The listing builds one solid part. Answer for the finished solid, in the listing's coordinates (mm). A direction names the side the tool comes from. Give positions to 0.01 mm unless a question says otherwise; leave off trailing zeros. Loops run counter-clockwise (first coordinate to the right, second up) from the corner with the lowest first, then second, coordinate; pieces in that order, holes last. Notation, with made-up numbers: (-9, -20.75) - (21, -20.75) arc R16 ccw to (21, -6.75) - close; hole circle Ø1 at (42.5, 42.5). An arc over 180 degrees is marked (long way). One line per item, written item: value. Start each with the question number.
Autodesk Fusion 360 part; units mm, degrees
sketch "Sketch1" plane through (0, 0, 0) normal (0, 0, 1) x (1, 0, 0)
  circle A0 centre (0, 0) radius 10
  dimension "d1" = 20
extrude "Extrude1" add sketch "Sketch1" along normal blind 3
sketch "Sketch2" plane through (0, 0, 3) normal (0, 0, 1) x (-1, 0, 0)
  circle A0 centre (0, 0) radius 10
  line L0 (-4.2, 1.3) -> (4.2, 1.3)
  line L1 (4.2, 1.3) -> (4.2, -1.3)
  line L2 (4.2, -1.3) -> (-4.2, -1.3)
  line L3 (-4.2, -1.3) -> (-4.2, 1.3)
  line L4 (-4.2, 1.3) -> (4.2, -1.3) construction
  line L5 (4.2, 1.3) -> (-4.2, -1.3) construction
  dimension "d4" = 8.4
  dimension "d5" = 2.6
extrude "Extrude2" cut sketch "Sketch2" against normal blind 6 contours L0 L1 L2 L3
fillet "Fillet1" radius 1.3 4 edges at (4.2, 1.3, 1.5) (4.2, -1.3, 1.5) (-4.2, 1.3, 1.5) (-4.2, -1.3, 1.5)
extrude "Extrude3" add 1 faces at (-0.2491, -4.1907, 3) along direction (0, 0, 1) blind 1
hole "Hole1" at (10, 0, 2.0667) direction (-1, 0, 0) diameter 2 depth 4 tip angle 180
mirror "Mirror1" about plane through (0, 0, 0) normal (1, 0, 0) of "Hole1"
1. A cutting plane is placed at D-D (y = -8.75). Determine the outline of the cut face in (x, z).
2. A cutting plane is placed at C-C (x = 8). Determine the outline of the cut face in (y, z).
3. Find the intervals of material crossed by L1, parallel to Z at x = 8, y = 0; L2, parallel to Y at x = 3.75, z = 1.2; L3, parallel to Y at x = -1.5, z = 0.7, in increasing order. Write a range as [from, to].
4. A cutting plane is placed at A-A (x = 0). Determine the outline of the cut face in (y, z), plus the area to 3 significant figures.
5. Determine the mould class of faces 1 (the flat face through (0, -2, 4)), 2 (the flat face through (-6, 0, 2)), 3 (the cylindrical face through (3.81, 0.93, 1.97)) for opening direction X: released by +X, released by -X, zero draft, split by the parting line, or undercut.
6. For faces 4 (the flat face through (0, -2, 0)), 5 (the cylindrical face through (3.83, -0.91, 1.97)), 6 (the flat face through (6, 0, 2)), 7 (the cylindrical face through (-7.97, -0.61, 2.86)), determine the directions among +Z, -Z, +X, -X, +Y, -Y from which every point of the face is accessible in a straight line to the end or side of a thin tool.
7. Flat-ended cylindrical pins translate along their axes: pin 1 (1 mm diameter, centred on y = -0.5, z = 1.5, fed in from +X); pin 2 (1.6 mm diameter, centred on y = 0, z = 2, fed in from -X); pin 3 (1.6 mm diameter, centred on y = 0, z = 2.07, fed in from +X). Find the tip coordinate at first contact, or state that the pin passes through.
Results below:
1. outline: (-4.84, 0) - (4.84, 0) - (4.84, 4) - (-4.84, 4) - close
2. outline: (-6, 0) - (6, 0) - (6, 4) - (-6, 4) - close; hole circle Ø2 at (0, 2.07)
3. L1: z = [0, 1.07], [3.07, 4]
3. L2: y = [-9.27, -0.98], [0.98, 9.27]
3. L3: y = [-9.89, -1.3], [1.3, 9.89]
4. outline: (-10, 0) - (-1.3, 0) - (-1.3, 4) - (-10, 4) - close; (1.3, 0) - (10, 0) - (10, 4) - (1.3, 4) - close
4. area: 69.6 mm^2
5. face 1: zero draft
5. face 2: released by -X
5. face 3: undercut
6. face 4: -Z, +X, -X, +Y, -Y
6. face 5: +Z, -Z
6. face 6: +X
6. face 7: -X
7. pin 1: stops at x = 10
7. pin 2: stops at x = -6
7. pin 3: stops at x = 6
